from build123d import *

# Parameters (mm, degrees)
F0_W     = 40
F0_H     = 7.5
F1_DEPTH = 15
F2_W     = 40
F2_H     = 9.25
F2_H_2   = 7.5
F3_DEPTH = 4


with BuildPart() as f1:
    # F0 (on Top) → F1 (new body)
    with BuildSketch(Plane.XY):
        Rectangle(F0_W, F0_H)
    extrude(amount=F1_DEPTH)

    # F2 (on face) → F3 (join)
    with BuildSketch(Plane.XY.offset(15)):
        with Locations((0, 8.375)):
            Rectangle(F2_W, F2_H)
        Rectangle(F2_W, F2_H_2)
        with Locations((0, -8.375)):
            Rectangle(F2_W, F2_H)
    extrude(amount=F3_DEPTH)


solid = f1.part
Build history of the part. All positions in model axes, mm. A direction names the side the tool comes from. Round coordinates to 2 decimals unless told otherwise and drop trailing zeros. Order: outer loops, then holes, each group sorted by start corner. A loop starts at its lowest first (then second) coordinate and runs counter-clockwise, first axis right, second up. Notation, with made-up numbers: M 58.25,29.5 L 84.25,29.5 A18 ccw 84.25,58.5 Z; hole C 18,87.25 d11. An arc over 180 degrees is marked long. Use CSV: the item, a comma, the result in double quotes. Start each with the question number.
(1) Cut at A-A on x = 11.5. List the corners of the cut face in (y, z).
(2) Flat gauge pins, fed straight in: P1, Ø2, axis at x = 12.5, z = 5, coming from the +Y side; P2, Ø5, axis at x = 13, z = 12, coming from the -Y side; P3, Ø4.5, axis at x = -7, y = 7.5, coming from the -Z side. Where does each tip first touch, or does it go through?
(3) Cut at C-C on y = -5.25. List the corners of the cut face in (x, z), then the cut area to 3 significant figures.
(4) Cut at B-B on z = 5.5. List the corners of the cut face in (x, y), then the cut area to 3 significant figures.
(5) Drill centre lines: probe 1 along Y at (x, z) = (14.5, 1.75); probe 2 along Z at (x, y) = (15, 7.75). Where is each one in solid material? Low to high.
(6) Tool access for faces 1 (the face through (0, -8, 15)), 2 (the face through (20, 0, 11)), 3 (the face through (0, 8, 15)): list every direction of +Z, -Z, +X, -X, +Y, -Y with a clear straight run to the whole face (end or side of a thin tool).
Findings:
1,outline,"M -13,15 L -3.75,15 L -3.75,0 L 3.75,0 L 3.75,15 L 13,15 L 13,19 L -13,19 Z"
2,P1,"stops at y = 3.75"
2,P2,"stops at y = -3.75"
2,P3,"stops at z = 15"
3,outline,"M -20,15 L 20,15 L 20,19 L -20,19 Z"
3,area,"160 mm^2"
4,outline,"M -20,-3.75 L 20,-3.75 L 20,3.75 L -20,3.75 Z"
4,area,"300 mm^2"
5,probe 1,"y = -3.75 to 3.75"
5,probe 2,"z = 15 to 19"
6,face 1,"-Z, +X, -X, -Y"
6,face 2,"+Z, -Z, +X, +Y, -Y"
6,face 3,"-Z, +X, -X, +Y"
